```python
from build123d import *

# Parameters (mm, degrees)
CROQUIS1_R              = 7.5
CROQUIS1_R_2            = 2
SALIENTE_EXTRUIR1_DEPTH = 9
CROQUIS2_R              = 4
CORTAR_EXTRUIR1_DEPTH   = 4.5


with BuildPart() as part:
    # Croquis1 → Saliente-Extruir1 (new body)
    with BuildSketch(Plane.XY):
        with BuildLine():
            Line((-25.5, 40), (25.5, 40))
            ThreePointArc((25.5, 40), (27.621320344, 39.121320344), (28.5, 37))
            Line((28.5, 37), (28.5, -40))
            Line((28.5, -40), (-28.5, -40))
            Line((-28.5, -40), (-28.5, 37))
            ThreePointArc((-28.5, 37), (-27.621320344, 39.121320344), (-25.5, 40))
        make_face()
        with Locations((0, 10)):
            Circle(CROQUIS1_R, mode=Mode.SUBTRACT)
        with Locations((10, -30)):
            Circle(CROQUIS1_R_2, mode=Mode.SUBTRACT)
        with Locations((-10, -30)):
            Circle(CROQUIS1_R_2, mode=Mode.SUBTRACT)
        with Locations((-23, 33)):
            Circle(CROQUIS1_R_2, mode=Mode.SUBTRACT)
        with Locations((-23, -14.5)):
            Circle(CROQUIS1_R_2, mode=Mode.SUBTRACT)
        with Locations(Location((23, -14.5, 0), (0, 0, 180))):
            Circle(CROQUIS1_R_2, mode=Mode.SUBTRACT)
        with Locations(Location((23, 33, 0), (0, 0, 180))):
            Circle(CROQUIS1_R_2, mode=Mode.SUBTRACT)
    extrude(amount=SALIENTE_EXTRUIR1_DEPTH)

    # Croquis2 → Cortar-Extruir1 (cut)
    with BuildSketch(Plane.XY.offset(9)):
        with Locations((-10, -30)):
            Circle(CROQUIS2_R)
        with Locations((10, -30)):
            Circle(CROQUIS2_R)
    extrude(amount=-CORTAR_EXTRUIR1_DEPTH, mode=Mode.SUBTRACT)


solid = part.part
```
Geometry check sheet. Reference: the model listing, model coordinates, mm. A direction names the side the tool comes from. Round coordinates to 2 decimals unless told otherwise and drop trailing zeros. Order: outer loops, then holes, each group sorted by start corner. A loop starts at its lowest first (then second) coordinate and runs counter-clockwise, first axis right, second up. Notation, with made-up numbers: M -7.75,-37 L 50.25,-37 A30 cw 50.25,2 Z; hole C -7,-7.5 d6. An arc over 180 degrees is marked long. Answer as CSV lines item,"result".
1) Gauge pin test, flat end, axial feed: pin 1 Ø2.5 at (x, y) = (9.5, -29) entering from +Z. Record the tip position at first contact, or that the pin passes through.
Entries:
pin 1,"z = 4.5"
2) Thickness scan on probe 1 along Y at (x, z) = (23, 6); probe 2 along X at (y, z) = (-30, 3.45); probe 3 along X at (y, z) = (10.5, 3.5). Record the ranges inside material, lowest first. Write a range as [from, to].
Entries:
probe 1,"[-40, -16.5], [-12.5, 31], [35, 40]"
probe 2,"[-28.5, -12], [-8, 8], [12, 28.5]"
probe 3,"[-28.5, -7.48], [7.48, 28.5]"
3) Tool access check on faces 1 (the face through (-9, -28, 4.5)), 2 (the face through (-23.26, -12.517, 4.437)). Record the directions out of +Z, -Z, +X, -X, +Y, -Y that give a thin tool (end or side, any length) a straight path to the whole face; none if there is none.
Entries:
face 1,"+Z"
face 2,"+Z, -Z"
4) Sectioned sample at B-B on z = 6.5. Record the cut outline in (x, y).
Entries:
outline,"M -28.5,-40 L 28.5,-40 L 28.5,37 A3 ccw 25.5,40 L -25.5,40 A3 ccw -28.5,37 Z; hole C -23,-14.5 d4; hole C -23,33 d4; hole C -10,-30 d8; hole C 0,10 d15; hole C 10,-30 d8; hole C 23,-14.5 d4; hole C 23,33 d4"
5) Mould release check, pull along X, two halves, no side actions. Record for faces 3 (the face through (27.6, 39.14, 4.44)), 4 (the face through (-1.63, 2.68, 4.44)), 5 (the face through (0, 1, 9)): +X half, -X half, draft (parallel to the pull), parting line (faces both ways), or undercut.
Entries:
face 3,"+X half"
face 4,"undercut"
face 5,"draft"
6) Sectioned sample at C-C on x = 0. Record the cut outline in (y, z), and give its area (3 significant figures).
Entries:
outline,"M -40,0 L 2.5,0 L 2.5,9 L -40,9 Z; M 17.5,0 L 40,0 L 40,9 L 17.5,9 Z"
area,"585 mm2"
7) Sectioned sample at A-A on x = 23. Record the cut outline in (y, z).
Entries:
outline,"M -40,0 L -16.5,0 L -16.5,9 L -40,9 Z; M -12.5,0 L 31,0 L 31,9 L -12.5,9 Z; M 35,0 L 40,0 L 40,9 L 35,9 Z"
8) Sectioned sample at D-D on x = 10. Record the cut outline in (y, z).
Entries:
outline,"M -40,0 L -32,0 L -32,4.5 L -34,4.5 L -34,9 L -40,9 Z; M -28,0 L 40,0 L 40,9 L -26,9 L -26,4.5 L -28,4.5 Z"
